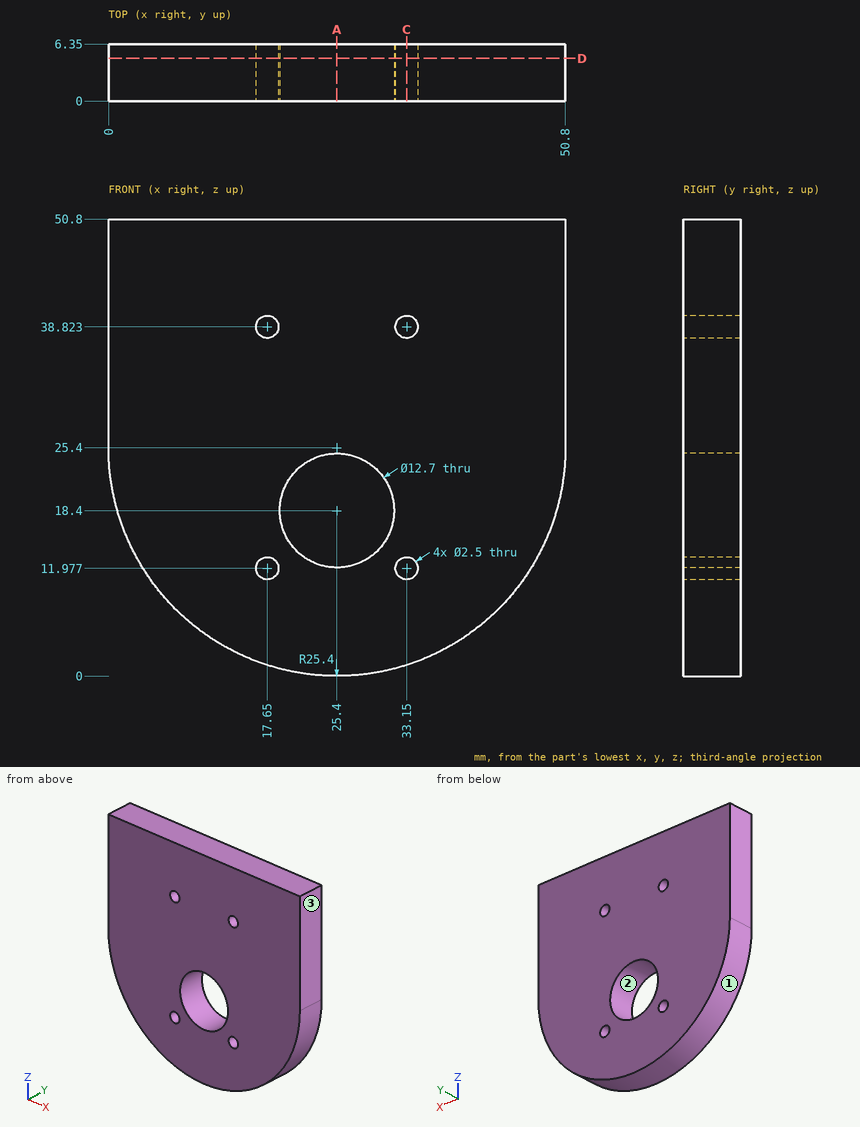
For this review, use the dimensioned drawing (mm, ordinates from the lowest corner) and the shaded views. Coordinates: 2 decimals unless noted, no trailing zeros. Loops run counter-clockwise (first coordinate to the right, second up) from the corner with the lowest first, then second, coordinate; pieces in that order, holes last. Notation, with made-up numbers: (69.5, 68) -> (82.5, 68) arc R25 cw to (82.5, 100) -> close; hole circle Ø7 at (77, -26.5). An arc over 180 degrees is marked (long way). Use a Markdown table: item, result. Add a question column.
1. Clearance check with flat-ended pins moving along their axes: pin 1 Ø2 at (x, z) = (33.15, 11.98) entering from +Y; pin 2 Ø1.5 at (x, y) = (31, 3.5) entering from -Z. State where each tip first meets the part, or that it passes through.
2. Draft analysis for pull direction Z (two halves, no side actions). For the marked faces 1, 2 and 3, state which applies: pulls with the +Z half, pulls with the -Z half, needs draft (parallel to the pull), parting line crosses it, or undercut.
3. Add section A-A on x = 25.4. Write out the cut boundary in (y, z), plus the area to 3 significant figures.
4. To check wall thickness, follow line 1 (X direction, y = 0.5, z = 11.5) (1 decimal); line 2 (Z direction, x = 25, y = 6.25); line 3 (Z direction, x = 17.65, y = 3.5). State the ranges of each line that lie inside material, in increasing order.
5. Add section D-D on y = 4.75. Write out the cut boundary in (x, z).
6. Add section C-C on x = 33.15. Write out the cut boundary in (y, z).
Returned:
| question | item | result |
|---|---|---|
| 1 | pin 1 | passes through |
| 1 | pin 2 | stops at z = 0.47 |
| 2 | face 1 | pulls with the -Z half |
| 2 | face 2 | undercut |
| 2 | face 3 | needs draft |
| 3 | outline | (0, 0) -> (6.35, 0) -> (6.35, 12.05) -> (0, 12.05) -> close; (0, 24.75) -> (6.35, 24.75) -> (6.35, 50.8) -> (0, 50.8) -> close |
| 3 | area | 242 mm² |
| 4 | line 1 | x = 4.1 to 16.5, 18.8 to 32, 34.3 to 46.7 |
| 4 | line 2 | z = 0 to 12.06, 24.74 to 50.8 |
| 4 | line 3 | z = 1.21 to 10.73, 13.23 to 37.57, 40.07 to 50.8 |
| 5 | outline | (0, 25.4) arc R25.4 ccw to (50.8, 25.4) -> (50.8, 50.8) -> (0, 50.8) -> close; hole circle Ø2.5 at (17.65, 11.98); hole circle Ø2.5 at (17.65, 38.82); hole circle Ø12.7 at (25.4, 18.4); hole circle Ø2.5 at (33.15, 11.98); hole circle Ø2.5 at (33.15, 38.82) |
| 6 | outline | (0, 1.21) -> (6.35, 1.21) -> (6.35, 10.73) -> (0, 10.73) -> close; (0, 13.23) -> (6.35, 13.23) -> (6.35, 37.57) -> (0, 37.57) -> close; (0, 40.07) -> (6.35, 40.07) -> (6.35, 50.8) -> (0, 50.8) -> close |
